Work out the finished part from the listing and answer in its coordinate system (mm). A direction names the side the tool comes from. Coordinates: 2 decimals unless noted, no trailing zeros. Order: outer loops, then holes, each group sorted by start corner. A loop starts at its lowest first (then second) coordinate and runs counter-clockwise, first axis right, second up. Notation, with made-up numbers: (51.5, 41) -> (59.5, 41) arc R25 cw to (59.5, 59) -> close; hole circle Ø10 at (40, 6). An arc over 180 degrees is marked (long way). Use one line per item in the form item = value.
from build123d import *

# Parameters (mm, degrees)
SALIENTE_EXTRUIR1_DEPTH      = 2.5
SALIENTE_EXTRUIR1_DEPTH_BACK = 2.5
CROQUIS2_R                   = 1.1
CORTAR_EXTRUIR1_DEPTH        = 7.123724357
REDONDEO1_R                  = 0.2
REDONDEO2_R                  = 0.2


with BuildPart() as part:
    # Croquis1 → Saliente-Extruir1 (new, two sides: drawn at the far end of the back side and taken through both)
    with BuildSketch(Plane.XY.offset(-SALIENTE_EXTRUIR1_DEPTH_BACK)):
        with BuildLine():
            Line((-5, 1.25), (0, 1.25))
            ThreePointArc((0, 1.25), (1.25, 0), (0, -1.25))
            Line((0, -1.25), (-5, -1.25))
            Line((-5, -1.25), (-5, -0.75))
            Line((-5, -0.75), (0, -0.75))
            ThreePointArc((0, -0.75), (0.75, 0), (0, 0.75))
            Line((0, 0.75), (-5, 0.75))
            Line((-5, 0.75), (-5, 1.25))
        make_face()
    extrude(amount=SALIENTE_EXTRUIR1_DEPTH + SALIENTE_EXTRUIR1_DEPTH_BACK)

    # Croquis2 → Cortar-Extruir1 (cut, through all)
    with BuildSketch(Plane(origin=(0, 1.25, 0), x_dir=(1, 0, 0), z_dir=(0, 1, 0))):
        with Locations(Location((-3, 0, 0), (0, 0, 270))):
            Circle(CROQUIS2_R)
        with BuildLine():
            ThreePointArc((-4.330785349, -2.5), (-4.820313987, -1.330516743), (-5, -0.075509846))
            Line((-5, -0.075509846), (-5, -2.5))
            Line((-5, -2.5), (-4.330785349, -2.5))
        make_face()
        with BuildLine():
            Line((-5, 2.5), (-5, 0.075509846))
            ThreePointArc((-5, 0.075509846), (-4.820313987, 1.330516743), (-4.330785349, 2.5))
            Line((-4.330785349, 2.5), (-5, 2.5))
        make_face()
    extrude(amount=-CORTAR_EXTRUIR1_DEPTH, mode=Mode.SUBTRACT)

    # Redondeo1
    redondeo1_edges = [part.edges().sort_by_distance(p)[0] for p in [
        (0.75, 0, 2.5),
        (-2.165392674, -0.75, 2.5),
        (1.25, 0, 2.5),
        (-2.165392674, 1.25, 2.5),
        (-2.165392674, 0.75, 2.5),
        (-2.165392674, -1.25, 2.5),
        (-4.330785349, 1, 2.5),
        (-4.330785349, -1, 2.5),
    ]]
    fillet(redondeo1_edges, radius=REDONDEO1_R)

    # Redondeo2
    redondeo2_edges = [part.edges().sort_by_distance(p)[0] for p in [
        (0.75, 0, -2.5),
        (-2.165392674, -0.75, -2.5),
        (1.25, 0, -2.5),
        (-2.165392674, 1.25, -2.5),
        (-2.165392674, -1.25, -2.5),
        (-2.165392674, 0.75, -2.5),
        (-4.330785349, 1, -2.5),
        (-4.330785349, -1, -2.5),
    ]]
    fillet(redondeo2_edges, radius=REDONDEO2_R)


solid = part.part
(1) Section C-C on y = 0 is taken. Write down the section's boundary in (x, z).
Data:
outline = (0.75, -2.3) arc R0.2 ccw to (0.95, -2.5) -> (1.05, -2.5) arc R0.2 ccw to (1.25, -2.3) -> (1.25, 2.3) arc R0.2 ccw to (1.05, 2.5) -> (0.95, 2.5) arc R0.2 ccw to (0.75, 2.3) -> close
(2) This flat-tipped pin is pushed along its axis until it touches: P1, Ø3, axis at x = -3, z = 0, coming from the +Y side. Where does it stop, or does it pass through?
Data:
P1 = 1.25
(3) Section A-A on z = 0 is taken. Write down the section's boundary in (x, y).
Data:
outline = (-5, -1.25) -> (-4.1, -1.25) -> (-4.1, -0.75) -> (-5, -0.75) -> close; (-5, 0.75) -> (-4.1, 0.75) -> (-4.1, 1.25) -> (-5, 1.25) -> close; (-1.9, -1.25) -> (0, -1.25) arc R1.25 ccw to (0, 1.25) -> (-1.9, 1.25) -> (-1.9, 0.75) -> (0, 0.75) arc R0.75 cw to (0, -0.75) -> (-1.9, -0.75) -> close
(4) Straight lines are drawn through the part: line 1 along Y through (x, z) = (-1, -1.15); line 2 along X through (y, z) = (0.95, 0); line 3 along X through (y, z) = (0.9, 0). For each, find the intervals that lie inside material, in ascending order.
Data:
line_1 = -1.25 to -0.75, 0.75 to 1.25
line_2 = -5 to -4.1, -1.9 to 0.81
line_3 = -5 to -4.1, -1.9 to 0.87
(5) The mould has two halves that part along Y. Classify faces 1 (the cylindrical face through (0.75, -0.02, -0.03)), 2 (the flat face through (-2, -0.75, -1)), 3 (the cylindrical face through (1.25, 0.03, -0.03)), 4 (the cylindrical face through (-4.074, 1.004, -0.238)): released by +Y, released by -Y, zero draft, split by the parting line, or undercut.
Data:
face_1 = undercut
face_2 = undercut
face_3 = split by the parting line
face_4 = zero draft
(6) Section D-D on x = -3 is taken. Write down the section's boundary in (y, z).
Data:
outline = (-1.25, -2.3) arc R0.2 ccw to (-1.05, -2.5) -> (-0.95, -2.5) arc R0.2 ccw to (-0.75, -2.3) -> (-0.75, -1.1) -> (-1.25, -1.1) -> close; (-1.25, 1.1) -> (-0.75, 1.1) -> (-0.75, 2.3) arc R0.2 ccw to (-0.95, 2.5) -> (-1.05, 2.5) arc R0.2 ccw to (-1.25, 2.3) -> close; (0.75, -2.3) arc R0.2 ccw to (0.95, -2.5) -> (1.05, -2.5) arc R0.2 ccw to (1.25, -2.3) -> (1.25, -1.1) -> (0.75, -1.1) -> close; (0.75, 1.1) -> (1.25, 1.1) -> (1.25, 2.3) arc R0.2 ccw to (1.05, 2.5) -> (0.95, 2.5) arc R0.2 ccw to (0.75, 2.3) -> close
(7) Section B-B on x = -1.75 is taken. Write down the section's boundary in (y, z), plus the area to 3 significant figures.
Data:
outline = (-1.25, -2.3) arc R0.2 ccw to (-1.05, -2.5) -> (-0.95, -2.5) arc R0.2 ccw to (-0.75, -2.3) -> (-0.75, 2.3) arc R0.2 ccw to (-0.95, 2.5) -> (-1.05, 2.5) arc R0.2 ccw to (-1.25, 2.3) -> close; (0.75, -2.3) arc R0.2 ccw to (0.95, -2.5) -> (1.05, -2.5) arc R0.2 ccw to (1.25, -2.3) -> (1.25, 2.3) arc R0.2 ccw to (1.05, 2.5) -> (0.95, 2.5) arc R0.2 ccw to (0.75, 2.3) -> close
area = 4.93 mm²
(8) Which of the six approach directions +Z, -Z, +X, -X, +Y, -Y give full straight-line access (tool end or side, diameter ignored) to faces 5 (the flat face through (-2, 0.75, -1)), 6 (the flat face through (-2, 1.25, -1))?
Data:
face_5 = +Z, -Z, -X
face_6 = +Z, -Z, +X, -X, +Y
